```python
from build123d import *

# Parameters (mm, degrees)
SKETCH1_W                                         = 23
SKETCH1_H                                         = 40.5
BOSS_EXTRUDE1_DEPTH                               = 10
CHAMBRAGE_POUR_VIS_SIX_PANS_CREUX_M61_D           = 6.6
CHAMBRAGE_POUR_VIS_SIX_PANS_CREUX_M61_CBORE_D     = 11
CHAMBRAGE_POUR_VIS_SIX_PANS_CREUX_M61_CBORE_DEPTH = 6.4
BOSS_EXTRUDE2_DEPTH                               = 2
ESQUISSE5_R                                       = 0.95
ENL_V_MAT_EXTRU_1_DEPTH                           = 4


with BuildPart() as part:
    # Sketch1 → Boss-Extrude1 (new body)
    with BuildSketch(Plane(origin=(0, 0, 0), x_dir=(0, 0, -1), z_dir=(1, 0, 0))):
        with Locations((0, -20.25)):
            Rectangle(SKETCH1_W, SKETCH1_H)
    extrude(amount=BOSS_EXTRUDE1_DEPTH)

    # Chambrage pour vis à six pans creux M61 (through all)
    with Locations(Plane(origin=(10, 0, 0), x_dir=(0, 0, -1), z_dir=(1, 0, 0))):
        with Locations((0, -30)):
            CounterBoreHole(CHAMBRAGE_POUR_VIS_SIX_PANS_CREUX_M61_D / 2, CHAMBRAGE_POUR_VIS_SIX_PANS_CREUX_M61_CBORE_D / 2, CHAMBRAGE_POUR_VIS_SIX_PANS_CREUX_M61_CBORE_DEPTH)

    # Sketch4 → Boss-Extrude2 (add)
    with BuildSketch(Plane.XY.offset(11.5)):
        with BuildLine():
            Line((10, 0), (18, 0))
            Line((18, 0), (18, 1.1))
            ThreePointArc((18, 1.1), (18.292893219, 1.807106781), (19, 2.1))
            Line((19, 2.1), (19.6, 2.1))
            ThreePointArc((19.6, 2.1), (20.307106781, 1.807106781), (20.6, 1.1))
            Line((20.6, 1.1), (20.6, -2))
            ThreePointArc((20.6, -2), (20.307106781, -2.707106781), (19.6, -3))
            Line((19.6, -3), (10, -3))
            Line((10, -3), (10, 0))
        make_face()
        with BuildLine():
            Line((10, -30.7), (18, -30.7))
            Line((18, -30.7), (18, -29.6))
            ThreePointArc((18, -29.6), (18.292893219, -28.892893219), (19, -28.6))
            Line((19, -28.6), (19.6, -28.6))
            ThreePointArc((19.6, -28.6), (20.307106781, -28.892893219), (20.6, -29.6))
            Line((20.6, -29.6), (20.6, -32.7))
            ThreePointArc((20.6, -32.7), (20.307106781, -33.407106781), (19.6, -33.7))
            Line((19.6, -33.7), (10, -33.7))
            Line((10, -33.7), (10, -30.7))
        make_face()
    boss_extrude2 = extrude(amount=-BOSS_EXTRUDE2_DEPTH)

    # Mirror1: Boss-Extrude2 across plane
    add(boss_extrude2.mirror(Plane.XY))

    # Esquisse5 → Enlèv. mat.-Extru.1 (cut)
    with BuildSketch(Plane.XY.offset(11.5)):
        with Locations((5, -5)):
            Circle(ESQUISSE5_R)
    enl_v_mat_extru_1 = extrude(amount=-ENL_V_MAT_EXTRU_1_DEPTH, mode=Mode.SUBTRACT)

    # Symétrie1: Enlèv. mat.-Extru.1 across plane
    add(enl_v_mat_extru_1.mirror(Plane.XY), mode=Mode.SUBTRACT)


solid = part.part
```
Part model, mm, in its own coordinate system. A direction names the side the tool comes from. Round coordinates to 2 decimals unless told otherwise and drop trailing zeros. Loops run counter-clockwise (first coordinate to the right, second up) from the corner with the lowest first, then second, coordinate; pieces in that order, holes last.
1. 3-axis set-ups, long thin cutter, end or side, ignore diameter. For faces 1 (the face through (15, -3, -11)), 2 (the face through (14, -30.7, -11)), 3 (the face through (15, -33.7, -11)): which of +Z, -Z, +X, -X, +Y, -Y reach the whole face in a straight line?
Solutions:
face 1: +Z, -Z, +X
face 2: +Z, -Z
face 3: +Z, -Z, +X, -Y
2. Two-plate mould, pull along Z, no slides. Class faces 4 (the face through (6.845, -24.547, 0.716)), 5 (the face through (5, -5, 7.5)), 6 (the face through (18.285, -28.901, 10.514)): pulls with the +Z half, pulls with the -Z half, needs draft (parallel to the pull), parting line crosses it, or undercut.
Solutions:
face 4: undercut
face 5: pulls with the +Z half
face 6: needs draft
3. Drill centre lines: line 1 along Z through (x, y) = (12.25, -2.5); line 2 along Y through (x, z) = (1.4, 0); line 3 along Y through (x, z) = (5, 8.4). Where is each one in solid material? Low to high.
Solutions:
line 1: z = -11.5 to -9.5, 9.5 to 11.5
line 2: y = -40.5 to -33.3, -26.7 to 0
line 3: y = -40.5 to -5.95, -4.05 to 0
4. Slice it at A-A (x = 5). Give the cut face in (y, z).
Solutions:
outline: (-40.5, -11.5) - (-5.95, -11.5) - (-5.95, -7.5) - (-4.05, -7.5) - (-4.05, -11.5) - (0, -11.5) - (0, 11.5) - (-4.05, 11.5) - (-4.05, 7.5) - (-5.95, 7.5) - (-5.95, 11.5) - (-40.5, 11.5) - close; hole circle Ø11 at (-30, 0)
5. Slice it at B-B (z = 0). Give the cut face in (x, y), and give its area (3 significant figures).
Solutions:
outline: (0, -40.5) - (10, -40.5) - (10, -35.5) - (3.6, -35.5) - (3.6, -33.3) - (0, -33.3) - close; (0, -26.7) - (3.6, -26.7) - (3.6, -24.5) - (10, -24.5) - (10, 0) - (0, 0) - close
area: 311 mm2
6. Slice it at C-C (x = 11). Give the cut face in (y, z).
Solutions:
outline: (-33.7, -11.5) - (-30.7, -11.5) - (-30.7, -9.5) - (-33.7, -9.5) - close; (-33.7, 9.5) - (-30.7, 9.5) - (-30.7, 11.5) - (-33.7, 11.5) - close; (-3, -11.5) - (0, -11.5) - (0, -9.5) - (-3, -9.5) - close; (-3, 9.5) - (0, 9.5) - (0, 11.5) - (-3, 11.5) - close
7. Flat gauge pins, fed straight in: pin 1 (12 mm diameter, centred on y = -18.5, z = -0.5, fed in from +X); pin 2 (1.5 mm diameter, centred on x = 5, y = -5, fed in from -Z); pin 3 (10 mm diameter, centred on y = -30, z = 0, fed in from +X). Where does each tip first touch, or does it go through?
Solutions:
pin 1: stops at x = 10
pin 2: stops at z = -7.5
pin 3: stops at x = 3.6
8. Slice it at D-D (y = -27.5). Give the cut face in (x, z).
Solutions:
outline: (0, -11.5) - (10, -11.5) - (10, -4.9) - (3.6, -4.9) - (3.6, -2.15) - (0, -2.15) - close; (0, 2.15) - (3.6, 2.15) - (3.6, 4.9) - (10, 4.9) - (10, 11.5) - (0, 11.5) - close
